Verification items for this drawing (mm, ordinates from the low corner). Round coordinates to 2 decimals unless told otherwise and drop trailing zeros. Write each loop counter-clockwise with the first axis right and the second up, starting at its lowest first coordinate (ties: lowest second). Pieces come first, ordered by that corner, then holes. Notation, with made-up numbers: (12.5, 70.5) -> (24.5, 70.5) arc R29 ccw to (24.5, 108.5) -> close; hole circle Ø1 at (58.25, -36). An arc over 180 degrees is marked (long way). One line per question, with ' | ' between items.
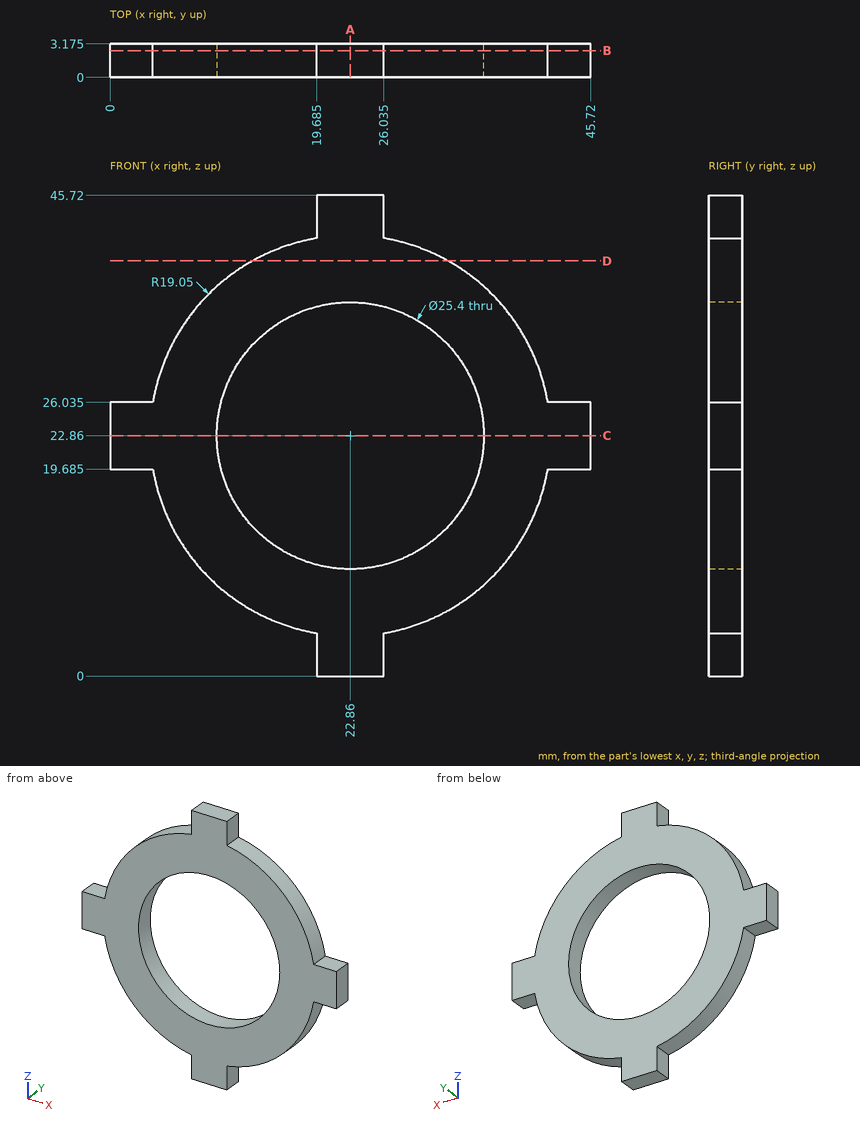
(1) Sectioned sample at D-D on z = 39.5. Record the cut outline in (x, y) (3 decimals), then the cut area to 3 significant figures.
Resolved:
outline: (13.586, 0) -> (32.134, 0) -> (32.134, 3.175) -> (13.586, 3.175) -> close | area: 58.9 mm2
(2) Sectioned sample at B-B on y = 2.55. Record the cut outline in (x, z) (3 decimals), then the cut area to 3 significant figures.
Resolved:
outline: (0, 19.685) -> (4.076, 19.685) arc R19.05 ccw to (19.685, 4.076) -> (19.685, 0) -> (26.035, 0) -> (26.035, 4.076) arc R19.05 ccw to (41.644, 19.685) -> (45.72, 19.685) -> (45.72, 26.035) -> (41.644, 26.035) arc R19.05 ccw to (26.035, 41.644) -> (26.035, 45.72) -> (19.685, 45.72) -> (19.685, 41.644) arc R19.05 ccw to (4.076, 26.035) -> (0, 26.035) -> close; hole circle Ø25.4 at (22.86, 22.86) | area: 732 mm2
(3) Sectioned sample at C-C on z = 22.86. Record the cut outline in (x, y) (3 decimals).
Resolved:
outline: (0, 0) -> (10.16, 0) -> (10.16, 3.175) -> (0, 3.175) -> close; (35.56, 0) -> (45.72, 0) -> (45.72, 3.175) -> (35.56, 3.175) -> close
(4) Sectioned sample at A-A on x = 22.86. Record the cut outline in (y, z) (3 decimals), then the cut area to 3 significant figures.
Resolved:
outline: (0, 0) -> (3.175, 0) -> (3.175, 10.16) -> (0, 10.16) -> close; (0, 35.56) -> (3.175, 35.56) -> (3.175, 45.72) -> (0, 45.72) -> close | area: 64.5 mm2
(5) Material ranges on line 1 (Z direction, x = 22.86, y = 2.2); line 2 (Z direction, x = 27.5, y = 3.05), recorded low to high.
Resolved:
line 1: z = 0 to 10.16, 35.56 to 45.72 | line 2: z = 4.38 to 11.04, 34.68 to 41.34
(6) Go/stop test with flat-tipped pins: pin 1 (1.6 mm diameter, centred on y = 2.5, z = 2.5, fed in from -X) (3 decimals); pin 2 (1 mm diameter, centred on x = 43.5, y = 1, fed in from +Z) (3 decimals); pin 3 (1.5 mm diameter, centred on x = 39, y = 2.5, fed in from +Z); pin 4 (8 mm diameter, centred on x = 34, z = 36.5, fed in from -Y). Record where each tip stops, or that it passes through.
Resolved:
pin 1: stops at x = 19.685 | pin 2: stops at z = 26.035 | pin 3: stops at z = 34.09 | pin 4: stops at y = 0
